Geometry check sheet. Reference: the model listing, model coordinates, mm. Face numbers are marked on the shaded views. Round coordinates to 2 decimals unless told otherwise and drop trailing zeros. Loops run counter-clockwise (first coordinate to the right, second up) from the corner with the lowest first, then second, coordinate; pieces in that order, holes last. Notation, with made-up numbers: (-39, 0.25) - (16, 0.25) arc R5 ccw to (16, 6.25) - close; hole circle Ø4 at (7, 23.25). An arc over 180 degrees is marked (long way). Write item = value, one per line.
```python
from build123d import *

# Parameters (mm, degrees)
F0_W         = 120
F0_H         = 95
F0_R         = 3
F0_R_2       = 1.65
F0_R_3       = 11
F1_DEPTH     = 8
F2_R         = 1.5
F3_SIZE      = 1.8
F4_T1_DEPTH  = 8
F4_T4_ANGLE  = 90
F4_T6_ANGLE  = 90
F4_T8_ANGLE  = 90
F4_T10_ANGLE = 90
F4_T12_ANGLE = 90
F4_T14_ANGLE = 90
F4_T16_ANGLE = 90
F4_T18_ANGLE = 90
F5_SIZE      = 0.5


# Not quite as in the source:
# - a fillet or chamfer that OpenCascade refuses, or shapes differently, is made with other operations: its cross-section is extruded or revolved along the edge and cut away or added


with BuildPart() as f1:
    # F0 (on Top) → F1 (new body)
    with BuildSketch(Plane.XY):
        with Locations((-21.1694301665, -8.1955979578)):
            Rectangle(F0_W, F0_H)
        with Locations((-71.1694301665, -45.6955979578)):
            Circle(F0_R, mode=Mode.SUBTRACT)
        with Locations((-46.1694301665, -45.6955979578)):
            Circle(F0_R, mode=Mode.SUBTRACT)
        with Locations((-21.1694301665, -45.6955979578)):
            Circle(F0_R, mode=Mode.SUBTRACT)
        with Locations((-71.1694301665, -20.6955979578)):
            Circle(F0_R, mode=Mode.SUBTRACT)
        with Locations((-43.6694301665, -20.6955979578)):
            Circle(F0_R_2, mode=Mode.SUBTRACT)
        with Locations((3.8305698335, -45.6955979578)):
            Circle(F0_R, mode=Mode.SUBTRACT)
        with Locations((28.8305698335, -45.6955979578)):
            Circle(F0_R, mode=Mode.SUBTRACT)
        with Locations((-18.6694301665, -20.6955979578)):
            Circle(F0_R_2, mode=Mode.SUBTRACT)
        with Locations((3.8305698335, -20.6955979578)):
            Circle(F0_R, mode=Mode.SUBTRACT)
        with Locations((28.8305698335, -20.6955979578)):
            Circle(F0_R, mode=Mode.SUBTRACT)
        with Locations((-71.1694301665, 4.3044020422)):
            Circle(F0_R, mode=Mode.SUBTRACT)
        with Locations((-31.1694301665, -8.1955979578)):
            Circle(F0_R_3, mode=Mode.SUBTRACT)
        with Locations((-43.6694301665, 4.3044020422)):
            Circle(F0_R_2, mode=Mode.SUBTRACT)
        with Locations((-71.1694301665, 29.3044020422)):
            Circle(F0_R, mode=Mode.SUBTRACT)
        with Locations((-46.1694301665, 29.3044020422)):
            Circle(F0_R, mode=Mode.SUBTRACT)
        with Locations((-21.1694301665, 29.3044020422)):
            Circle(F0_R, mode=Mode.SUBTRACT)
        with Locations((-18.6694301665, 4.3044020422)):
            Circle(F0_R_2, mode=Mode.SUBTRACT)
        with Locations((3.8305698335, 4.3044020422)):
            Circle(F0_R, mode=Mode.SUBTRACT)
        with Locations((28.8305698335, 4.3044020422)):
            Circle(F0_R, mode=Mode.SUBTRACT)
        with Locations((3.8305698335, 29.3044020422)):
            Circle(F0_R, mode=Mode.SUBTRACT)
        with Locations((28.8305698335, 29.3044020422)):
            Circle(F0_R, mode=Mode.SUBTRACT)
    extrude(amount=-F1_DEPTH)

    # F2
    f2_edges = [f1.edges().sort_by_distance(p)[0] for p in [
        (-21.16943, -55.695598, 0),
        (38.83057, -8.195598, 0),
        (-21.16943, 39.304402, 0),
        (-81.16943, -8.195598, 0),
        (-21.16943, -55.695598, -8),
        (38.83057, -8.195598, -8),
        (-81.16943, -8.195598, -8),
        (-21.16943, 39.304402, -8),
    ]]
    fillet(f2_edges, radius=F2_R)

    # F3
    f3_edges = [f1.edges().sort_by_distance(p)[0] for p in [
        (-45.31943, 4.304402, 0),
        (-20.31943, 4.304402, 0),
        (-20.31943, -20.695598, 0),
        (-45.31943, -20.695598, 0),
        (-45.31943, -20.695598, -8),
        (-20.31943, 4.304402, -8),
        (-20.31943, -20.695598, -8),
        (-45.31943, 4.304402, -8),
    ]]
    chamfer(f3_edges, length=F3_SIZE)

    # F4: fillet of radius 3 on 4 edges, made by hand

    # F4_s2 → F4_t1 (cut)
    with BuildSketch(Plane.XY.offset(-8)):
        with BuildLine():
            ThreePointArc((-78.1694301665, -55.6955979578), (-80.29075051, -54.8169183014), (-81.1694301665, -52.6955979578))
            Line((-81.1694301665, -52.6955979578), (-81.1694301665, -55.6955979578))
            Line((-81.1694301665, -55.6955979578), (-78.1694301665, -55.6955979578))
        make_face()
        with BuildLine():
            ThreePointArc((35.8305698335, -55.6955979578), (37.9518901771, -54.8169183014), (38.8305698335, -52.6955979578))
            Line((38.8305698335, -52.6955979578), (38.8305698335, -55.6955979578))
            Line((38.8305698335, -55.6955979578), (35.8305698335, -55.6955979578))
        make_face()
        with BuildLine():
            ThreePointArc((-81.1694301665, 36.3044020422), (-80.29075051, 38.4257223857), (-78.1694301665, 39.3044020422))
            Line((-78.1694301665, 39.3044020422), (-81.1694301665, 39.3044020422))
            Line((-81.1694301665, 39.3044020422), (-81.1694301665, 36.3044020422))
        make_face()
        with BuildLine():
            ThreePointArc((38.8305698335, 36.3044020422), (37.9518901771, 38.4257223857), (35.8305698335, 39.3044020422))
            Line((35.8305698335, 39.3044020422), (38.8305698335, 39.3044020422))
            Line((38.8305698335, 39.3044020422), (38.8305698335, 36.3044020422))
        make_face()
    extrude(amount=F4_T1_DEPTH, mode=Mode.SUBTRACT)

    # F4_s3 → F4_t4 (revolve, cut)
    with BuildSketch(Plane.XZ.offset(-36.3044020422)):
        with BuildLine():
            ThreePointArc((37.3305698335, 0), (38.3912300053, -0.4393398282), (38.8305698335, -1.5))
            Line((38.8305698335, -1.5), (38.8305698335, 0))
            Line((38.8305698335, 0), (37.3305698335, 0))
        make_face()
    revolve(axis=Axis((35.8305698335, 36.3044020422, 0), (0, 0, 1)), revolution_arc=F4_T4_ANGLE, mode=Mode.SUBTRACT)

    # F4_s5 → F4_t6 (revolve, cut)
    with BuildSketch(Plane.YZ.offset(35.8305698335)):
        with BuildLine():
            ThreePointArc((37.8044020422, -8), (38.865062214, -7.5606601718), (39.3044020422, -6.5))
            Line((39.3044020422, -6.5), (39.3044020422, -8))
            Line((39.3044020422, -8), (37.8044020422, -8))
        make_face()
    revolve(axis=Axis((35.8305698335, 36.3044020422, -8), (0, 0, -1)), revolution_arc=F4_T6_ANGLE, mode=Mode.SUBTRACT)

    # F4_s7 → F4_t8 (revolve, cut)
    with BuildSketch(Plane.YZ.offset(-78.1694301665)):
        with BuildLine():
            ThreePointArc((37.8044020422, 0), (38.865062214, -0.4393398282), (39.3044020422, -1.5))
            Line((39.3044020422, -1.5), (39.3044020422, 0))
            Line((39.3044020422, 0), (37.8044020422, 0))
        make_face()
    revolve(axis=Axis((-78.1694301665, 36.3044020422, 0), (0, 0, 1)), revolution_arc=F4_T8_ANGLE, mode=Mode.SUBTRACT)

    # F4_s9 → F4_t10 (revolve, cut)
    with BuildSketch(Plane.XZ.offset(-36.3044020422)):
        with BuildLine():
            ThreePointArc((-79.6694301665, -8), (-80.7300903383, -7.5606601718), (-81.1694301665, -6.5))
            Line((-81.1694301665, -6.5), (-81.1694301665, -8))
            Line((-81.1694301665, -8), (-79.6694301665, -8))
        make_face()
    revolve(axis=Axis((-78.1694301665, 36.3044020422, -8), (0, 0, -1)), revolution_arc=F4_T10_ANGLE, mode=Mode.SUBTRACT)

    # F4_s11 → F4_t12 (revolve, cut)
    with BuildSketch(Plane.YZ.offset(35.8305698335)):
        with BuildLine():
            ThreePointArc((-54.1955979578, 0), (-55.2562581296, -0.4393398282), (-55.6955979578, -1.5))
            Line((-55.6955979578, -1.5), (-55.6955979578, 0))
            Line((-55.6955979578, 0), (-54.1955979578, 0))
        make_face()
    revolve(axis=Axis((35.8305698335, -52.6955979578, 0), (0, 0, 1)), revolution_arc=F4_T12_ANGLE, mode=Mode.SUBTRACT)

    # F4_s13 → F4_t14 (revolve, cut)
    with BuildSketch(Plane.XZ.offset(52.6955979578)):
        with BuildLine():
            ThreePointArc((37.3305698335, -8), (38.3912300053, -7.5606601718), (38.8305698335, -6.5))
            Line((38.8305698335, -6.5), (38.8305698335, -8))
            Line((38.8305698335, -8), (37.3305698335, -8))
        make_face()
    revolve(axis=Axis((35.8305698335, -52.6955979578, -8), (0, 0, -1)), revolution_arc=F4_T14_ANGLE, mode=Mode.SUBTRACT)

    # F4_s15 → F4_t16 (revolve, cut)
    with BuildSketch(Plane.XZ.offset(52.6955979578)):
        with BuildLine():
            ThreePointArc((-79.6694301665, 0), (-80.7300903383, -0.4393398282), (-81.1694301665, -1.5))
            Line((-81.1694301665, -1.5), (-81.1694301665, 0))
            Line((-81.1694301665, 0), (-79.6694301665, 0))
        make_face()
    revolve(axis=Axis((-78.1694301665, -52.6955979578, 0), (0, 0, 1)), revolution_arc=F4_T16_ANGLE, mode=Mode.SUBTRACT)

    # F4_s17 → F4_t18 (revolve, cut)
    with BuildSketch(Plane.YZ.offset(-78.1694301665)):
        with BuildLine():
            ThreePointArc((-54.1955979578, -8), (-55.2562581296, -7.5606601718), (-55.6955979578, -6.5))
            Line((-55.6955979578, -6.5), (-55.6955979578, -8))
            Line((-55.6955979578, -8), (-54.1955979578, -8))
        make_face()
    revolve(axis=Axis((-78.1694301665, -52.6955979578, -8), (0, 0, -1)), revolution_arc=F4_T18_ANGLE, mode=Mode.SUBTRACT)

    # F5
    f5_edges = [f1.edges().sort_by_distance(p)[0] for p in [
        (-74.16943, -45.695598, -8),
        (-74.16943, -45.695598, 0),
        (25.83057, -45.695598, -8),
        (0.83057, -45.695598, -8),
        (-49.16943, -45.695598, -8),
        (-24.16943, -45.695598, -8),
        (0.83057, -45.695598, 0),
        (25.83057, -45.695598, 0),
        (-24.16943, -45.695598, 0),
        (-49.16943, -45.695598, 0),
        (25.83057, 4.304402, -8),
        (0.83057, 4.304402, -8),
        (0.83057, -20.695598, -8),
        (0.83057, 4.304402, 0),
        (25.83057, -20.695598, -8),
        (25.83057, 29.304402, -8),
        (0.83057, -20.695598, 0),
        (0.83057, 29.304402, -8),
        (25.83057, 4.304402, 0),
        (0.83057, 29.304402, 0),
        (25.83057, 29.304402, 0),
        (25.83057, -20.695598, 0),
        (-24.16943, 29.304402, -8),
        (-49.16943, 29.304402, -8),
        (-74.16943, 29.304402, -8),
        (-24.16943, 29.304402, 0),
        (-49.16943, 29.304402, 0),
        (-74.16943, 29.304402, 0),
        (-74.16943, 4.304402, -8),
        (-74.16943, -20.695598, -8),
        (-74.16943, -20.695598, 0),
        (-74.16943, 4.304402, 0),
    ]]
    chamfer(f5_edges, length=F5_SIZE)


solid = f1.part
```
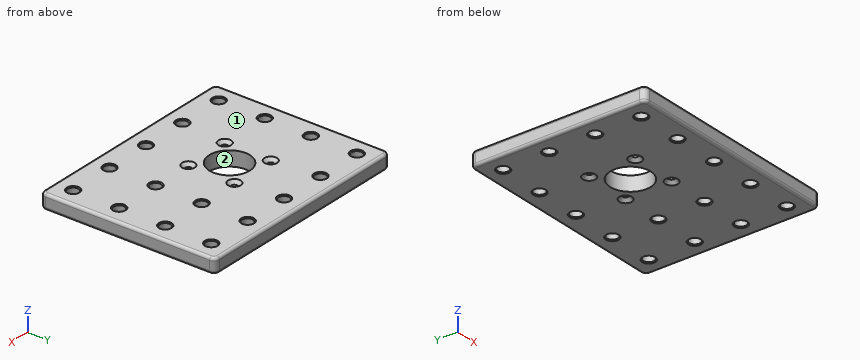
(1) Section check A-A (y = -6). Enter the section's corners in (x, z).
Answers follow:
outline = (-81.17, -6.5) arc R1.5 ccw to (-79.67, -8) - (-41.95, -8) - (-41.95, 0) - (-79.67, 0) arc R1.5 ccw to (-81.17, -1.5) - close; (-20.39, -8) - (37.33, -8) arc R1.5 ccw to (38.83, -6.5) - (38.83, -1.5) arc R1.5 ccw to (37.33, 0) - (-20.39, 0) - close
(2) Mould release check, pull along X, two halves, no side actions. Record for the marked faces 1 and 2: pulls with the +X half, pulls with the -X half, needs draft (parallel to the pull), parting line crosses it, or undercut.
Answers follow:
face_1 = needs draft
face_2 = undercut
(3) Gauge pin test, flat ends, axial feed: pin 1 (5.5 mm diameter, centred on x = -18.67, y = 4.3, fed in from -Z); pin 2 (4 mm diameter, centred on x = -43.67, y = 4.3, fed in from +Z). Record the tip position at first contact, or that the pin passes through.
Answers follow:
pin_1 = -7.3
pin_2 = -1.45
(4) Scan lines: L1, parallel to Y at x = -71, z = -4.5; L2, parallel to X at y = -46, z = -1.75; L3, parallel to X at y = 4, z = -5. Record each from-to range of solid material in increasing order. Write a range as [from, to].
Answers follow:
L1 = [-55.7, -48.69], [-42.7, -23.69], [-17.7, 1.31], [7.3, 26.31], [32.3, 39.3]
L2 = [-81.17, -74.15], [-68.18, -49.15], [-43.18, -24.15], [-18.18, 0.85], [6.82, 25.85], [31.82, 38.83]
L3 = [-81.17, -74.15], [-68.18, -45.29], [-42.05, -20.29], [-17.05, 0.85], [6.82, 25.85], [31.82, 38.83]
(5) Section check B-B (z = -4). State how many separate pieces and enclosed holes the cut face has, then the cut area to 3 significant figures.
Answers follow:
separate_pieces = 1
enclosed_holes = 21
area = 10,500 mm²
